```python
from build123d import *

# Parameters (mm, degrees)
SKETCH1_W           = 203.2
SKETCH1_H           = 80.772
BOSS_EXTRUDE1_DEPTH = 6.35
SKETCH2_R           = 2.5527
CUT_EXTRUDE1_DEPTH  = 8.89
CUT_EXTRUDE2_DEPTH  = 13.97
FILLET1_R           = 5.08


with BuildPart() as part:
    # Sketch1 → Boss-Extrude1 (new body)
    with BuildSketch(Plane.XY):
        with Locations((27.262808983, 8.108009164)):
            Rectangle(SKETCH1_W, SKETCH1_H)
    extrude(amount=BOSS_EXTRUDE1_DEPTH)

    # Sketch2 → Cut-Extrude1 (cut)
    with BuildSketch(Plane.XY.offset(6.35)):
        with Locations((-67.987191017, 42.144009164)):
            Circle(SKETCH2_R)
        with Locations((-67.987191017, -25.927990836)):
            Circle(SKETCH2_R)
        with Locations((122.512808983, 42.144009164)):
            Circle(SKETCH2_R)
        with Locations((122.512808983, -25.927990836)):
            Circle(SKETCH2_R)
    extrude(amount=-CUT_EXTRUDE1_DEPTH, mode=Mode.SUBTRACT)

    # Sketch3 → Cut-Extrude2 (cut)
    with BuildSketch(Plane.XY.offset(6.35)):
        with BuildLine():
            Line((-48.937191017, 36.147533789), (103.462808983, 36.147533789))
            ThreePointArc((103.462808983, 36.147533789), (106.102333608, 33.508009164), (103.462808983, 30.868484538))
            Line((103.462808983, 30.868484538), (-48.937191017, 30.868484538))
            ThreePointArc((-48.937191017, 30.868484538), (-51.576715642, 33.508009164), (-48.937191017, 36.147533789))
        make_face()
        with BuildLine():
            Line((-48.937191017, -14.449425855), (103.462808983, -14.449425855))
            ThreePointArc((103.462808983, -14.449425855), (106.305373964, -17.291990836), (103.462808983, -20.134555817))
            Line((103.462808983, -20.134555817), (-48.937191017, -20.134555817))
            ThreePointArc((-48.937191017, -20.134555817), (-51.779755998, -17.291990836), (-48.937191017, -14.449425855))
        make_face()
        with BuildLine():
            Line((-48.937191017, -6.829425855), (103.462808983, -6.829425855))
            ThreePointArc((103.462808983, -6.829425855), (105.258860207, -6.08547708), (106.002808983, -4.289425855))
            Line((106.002808983, -4.289425855), (106.002808983, 20.69451567))
            ThreePointArc((106.002808983, 20.69451567), (105.258860207, 22.490566894), (103.462808983, 23.23451567))
            Line((103.462808983, 23.23451567), (-48.937191017, 23.23451567))
            ThreePointArc((-48.937191017, 23.23451567), (-50.733242241, 22.490566894), (-51.477191017, 20.69451567))
            Line((-51.477191017, 20.69451567), (-51.477191017, -4.289425855))
            ThreePointArc((-51.477191017, -4.289425855), (-50.733242241, -6.08547708), (-48.937191017, -6.829425855))
        make_face()
    extrude(amount=-CUT_EXTRUDE2_DEPTH, mode=Mode.SUBTRACT)

    # Fillet1
    fillet1_edges = [part.edges().sort_by_distance(p)[0] for p in [
        (-74.337191017, 48.494009164, 3.175),
        (128.862808983, 48.494009164, 3.175),
        (128.862808983, -32.277990836, 3.175),
        (-74.337191017, -32.277990836, 3.175),
    ]]
    fillet(fillet1_edges, radius=FILLET1_R)


solid = part.part
```
The model under review builds one solid part; all positions refer to its coordinate system, in mm. A direction names the side the tool comes from. Coordinates: 2 decimals unless noted, no trailing zeros. Write each loop counter-clockwise with the first axis right and the second up, starting at its lowest first coordinate (ties: lowest second). Pieces come first, ordered by that corner, then holes. Notation, with made-up numbers: (-36.75, -10.75) - (15.25, -10.75) arc R19 ccw to (15.25, 11.25) - close; hole circle Ø1 at (10, -38.75). An arc over 180 degrees is marked (long way). Answer in a Markdown table with one row per item. Add a question column.
Q1. To check wall thickness, follow line 1 along Y through (x, z) = (44, 0.75); line 2 along X through (y, z) = (3, 5.25); line 3 along X through (y, z) = (33.5, 5). State the ranges of each line that lie inside material, in increasing order. Write a range as from..to.
Q2. Consider section B-B on x = 78. Give the boundary of the cut face in (y, z), then the cut area to 3 significant figures.
Q3. Clearance check with a flat-ended pin moving along its axis: pin 1 (12 mm diameter, centred on x = 77, y = 31.5, fed in from -Z). State where the tip first meets the part, or that it passes through.
Q4. Consider section C-C on z = 5. Give the boundary of the cut face in (x, y), then the cut area to 3 significant figures.
Q5. For faces 1 (the face through (127.335, 47.045, 3.219)), 2 (the face through (26, -6.829, 3)), list the 3-axis set-ups (+Z, -Z, +X, -X, +Y, -Y) from which the entire face can be reached by the end or side of a thin tool; tool diameter is ignored.
Q6. Consider section A-A on y = 1.5. Give the boundary of the cut face in (x, z).
Q7. Draft analysis for pull direction Y (two halves, no side actions). For faces 3 (the face through (-72.89, -30.75, 3.22)), 4 (the face through (106.1, 33.6, 3.2)), 5 (the face through (26, 48.494, 3)), state which applies: +Y half, -Y half, draft (parallel to the pull), parting line (faces both ways), or undercut.
Answers below:
| question | item | result |
|---|---|---|
| 1 | line 1 | -32.28..-20.13, -14.45..-6.83, 23.23..30.87, 36.15..48.49 |
| 1 | line 2 | -74.34..-51.48, 106..128.86 |
| 1 | line 3 | -74.34..-51.58, 106.1..128.86 |
| 2 | outline | (-32.28, 0) - (-20.13, 0) - (-20.13, 6.35) - (-32.28, 6.35) - close; (-14.45, 0) - (-6.83, 0) - (-6.83, 6.35) - (-14.45, 6.35) - close; (23.23, 0) - (30.87, 0) - (30.87, 6.35) - (23.23, 6.35) - close; (36.15, 0) - (48.49, 0) - (48.49, 6.35) - (36.15, 6.35) - close |
| 2 | area | 252 mm² |
| 3 | pin 1 | z = 0 |
| 4 | outline | (-74.34, -27.2) arc R5.08 ccw to (-69.26, -32.28) - (123.78, -32.28) arc R5.08 ccw to (128.86, -27.2) - (128.86, 43.41) arc R5.08 ccw to (123.78, 48.49) - (-69.26, 48.49) arc R5.08 ccw to (-74.34, 43.41) - close; hole circle Ø5.11 at (-67.99, -25.93); hole circle Ø5.11 at (-67.99, 42.14); hole (-51.48, -4.29) arc R2.54 ccw to (-48.94, -6.83) - (103.46, -6.83) arc R2.54 ccw to (106, -4.29) - (106, 20.69) arc R2.54 ccw to (103.46, 23.23) - (-48.94, 23.23) arc R2.54 ccw to (-51.48, 20.69) - close; hole (-48.94, -20.13) - (103.46, -20.13) arc R2.84 ccw to (103.46, -14.45) - (-48.94, -14.45) arc R2.84 ccw to start; hole (-48.94, 30.87) - (103.46, 30.87) arc R2.64 ccw to (103.46, 36.15) - (-48.94, 36.15) arc R2.64 ccw to start; hole circle Ø5.11 at (122.51, -25.93); hole circle Ø5.11 at (122.51, 42.14) |
| 4 | area | 9,860 mm² |
| 5 | face 1 | +Z, -Z, +X, +Y |
| 5 | face 2 | +Z, -Z |
| 6 | outline | (-74.34, 0) - (-51.48, 0) - (-51.48, 6.35) - (-74.34, 6.35) - close; (106, 0) - (128.86, 0) - (128.86, 6.35) - (106, 6.35) - close |
| 7 | face 3 | -Y half |
| 7 | face 4 | undercut |
| 7 | face 5 | +Y half |
